Source: three-view drawing plus pictorial views. Frame: mm from the lowest corner of the part. A direction names the side the tool comes from. Give positions to 0.01 mm unless a question says otherwise; leave off trailing zeros. Order: outer loops, then holes, each group sorted by start corner. A loop starts at its lowest first (then second) coordinate and runs counter-clockwise, first axis right, second up. Notation, with made-up numbers: (67.25, 80) - (85.25, 80) arc R22 ccw to (85.25, 98) - close; hole circle Ø5 at (66, 28.25). An arc over 180 degrees is marked (long way). Answer in a Markdown table with one row per item. Add a question column.
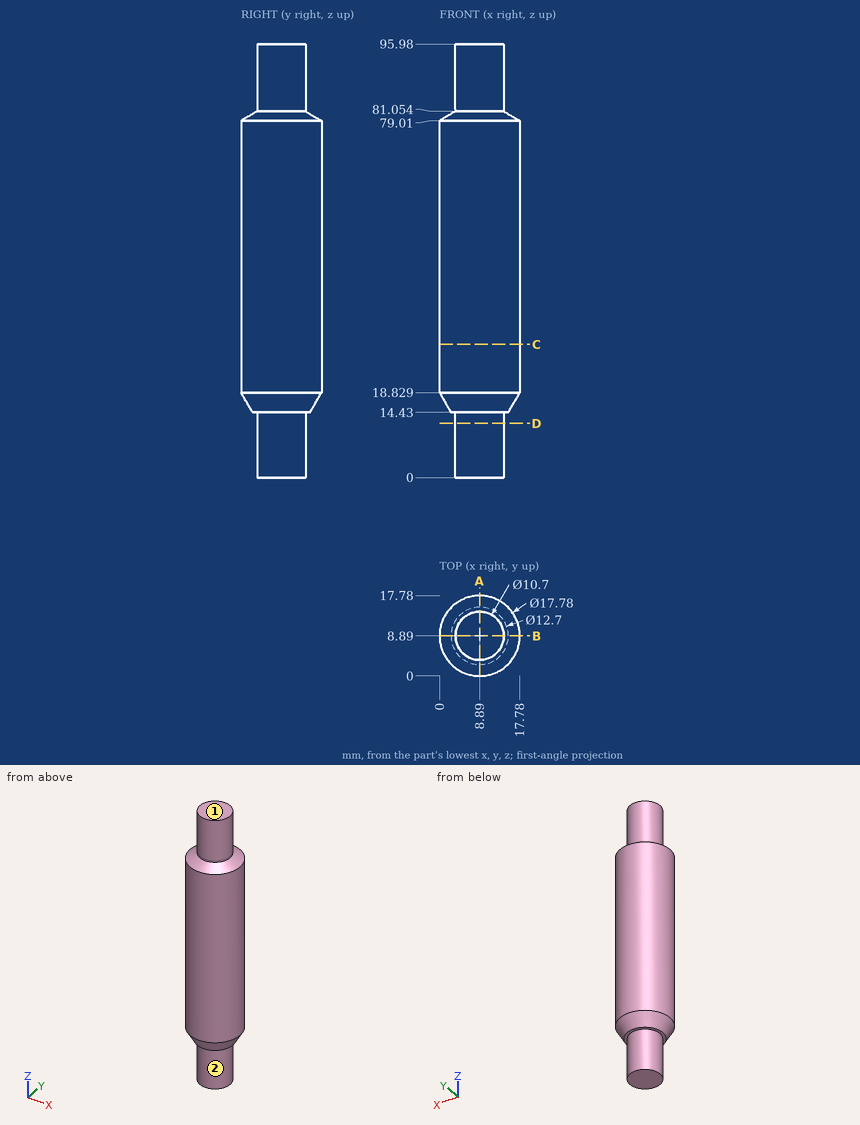
Q1. Section D-D, the plane z = 12. Return loops of the section in (x, y).
Q2. Line query: probe 1 along Y at (x, z) = (13.25, 51.5); probe 2 along X at (y, z) = (16.75, 73.5) (1 decimal); probe 3 along Y at (x, z) = (15, 51.5). Output: solid intervals per line, ascending.
Q3. Section C-C, the plane z = 29.5. Return loops of the section in (x, y).
Q4. Contact query for flat-ended pins moving along their axis: P1, Ø6, axis at x = 11.5, y = 4, coming from the +Z side; P2, Ø2, axis at x = 5, z = 43, coming from the -Y side; P3, Ø1, axis at x = 15.5, z = 11.5, coming from the -Y side; P4, Ø6, axis at y = 14.5, z = 13.5, coming from the +X side. Output: stop coordinate, or through.
Q5. Access query for the marked faces 1 and 2. Directions: +Z, -Z, +X, -X, +Y, -Y. A direction counts if a zero-diameter tool reaches every point of the face in a straight line with its end or side. Return the directions, or none.
Q6. Section A-A, the plane x = 8.89. Return loops of the section in (y, z), then the cut area to 3 significant figures.
Computed:
| question | item | result |
|---|---|---|
| 1 | outline | circle Ø10.7 at (8.89, 8.89) |
| 2 | probe 1 | y = 1.14 to 16.64 |
| 2 | probe 2 | x = 4.7 to 13 |
| 2 | probe 3 | y = 2.43 to 15.35 |
| 3 | outline | circle Ø17.78 at (8.89, 8.89) |
| 4 | P1 | stops at z = 95.98 |
| 4 | P2 | stops at y = 0.48 |
| 4 | P3 | passes through |
| 4 | P4 | stops at x = 15.01 |
| 5 | face 1 | +Z, +X, -X, +Y, -Y |
| 5 | face 2 | -Z |
| 6 | outline | (0, 18.83) - (2.54, 14.43) - (3.54, 14.43) - (3.54, 0) - (14.24, 0) - (14.24, 14.43) - (15.24, 14.43) - (17.78, 18.83) - (17.78, 79.01) - (14.24, 81.05) - (14.24, 95.98) - (3.54, 95.98) - (3.54, 81.05) - (0, 79.01) - close |
| 6 | area | 1,480 mm^2 |
